The model under review builds one solid part; all positions refer to its coordinate system, in mm. A direction names the side the tool comes from. Round coordinates to 2 decimals unless told otherwise and drop trailing zeros. Order: outer loops, then holes, each group sorted by start corner. A loop starts at its lowest first (then second) coordinate and runs counter-clockwise, first axis right, second up.
1) Consider section A-A (z = -3.2). Give the boundary of the cut face in (x, y).
2) Mouldability with a two-part tool opening along X and no side actions: class faces 1 (the face through (6.506, 0.072, -0.986)), 2 (the face through (-17.922, -9.404, -2.416)), 3 (the face through (-14, -9, -4)) as pulls with the +X half, pulls with the -X half, needs draft (parallel to the pull), parting line crosses it, or undercut.
3) Clearance check with flat-ended pins moving along their axes: P1, Ø1.5, axis at x = 4.5, z = -3, coming from the +Y side; P2, Ø12, axis at x = -6.5, y = 8, coming from the -Z side; P3, Ø1.5, axis at y = 0.5, z = -1, coming from the -X side. State where each tip first meets the part, or that it passes through.
4) Consider section D-D (x = -2). Give the boundary of the cut face in (y, z).
5) Consider section B-B (y = 7.7). Give the boundary of the cut face in (x, z).
6) Machinability: for faces 4 (the face through (6, -4.9, -1)), 5 (the face through (18.286, 6.628, -2.416)), 6 (the face through (0, -10.5, -1)), 7 (the face through (-6, 4.9, -1)), which of the approach directions +Z, -Z, +X, -X, +Y, -Y give a long, thin tool a straight path to every point of the face, cutting with its end or side? Answer none if there is none.
7) To check wall thickness, follow L1, parallel to Y at x = 15.7, z = -2.7; L2, parallel to Y at x = -15.7, z = -2.5; L3, parallel to Z at x = -2, y = 0.5. State the ranges of each line that lie inside material, in increasing order.
8) Consider section C-C (x = 11). Give the boundary of the cut face in (y, z).
from build123d import *

# Parameters (mm, degrees)
EXTRUDE_1007_DEPTH = 2
SKETCH_1_5_R       = 2.8
SKETCH_1_5_R_2     = 1.7
EXTRUDE_1109_DEPTH = 4


with BuildPart() as part:
    # Эскиз1 → Extrude 1007 (new body)
    with BuildSketch(Plane.XY):
        with BuildLine():
            Line((15.7, 10.5), (-15.7, 10.5))
            ThreePointArc((-15.7, 10.5), (-13.720101013, 9.679898987), (-12.9, 7.7))
            ThreePointArc((-12.9, 7.7), (-13.720101013, 5.720101013), (-15.7, 4.9))
            Line((-15.7, 4.9), (3.632157719, 4.9))
            Line((3.632157719, 4.9), (-16.932946461, -5.186070203))
            ThreePointArc((-16.932946461, -5.186070203), (-14.218826494, -5.323842378), (-12.9, -7.7))
            ThreePointArc((-12.9, -7.7), (-13.720101013, -9.679898987), (-15.7, -10.5))
            Line((-15.7, -10.5), (15.7, -10.5))
            ThreePointArc((15.7, -10.5), (12.9, -7.7), (15.7, -4.9))
            Line((15.7, -4.9), (-3.632157719, -4.9))
            Line((-3.632157719, -4.9), (16.932946461, 5.186070203))
            ThreePointArc((16.932946461, 5.186070203), (12.972455002, 7.067150662), (15.7, 10.5))
        make_face()
    extrude(amount=-EXTRUDE_1007_DEPTH)

    # Эскиз1<5> → Extrude 1109 (add)
    # profile 1 of 4: a face of its own
    with BuildSketch(Plane.XY):
        with Locations((15.7, 7.7)):
            Circle(SKETCH_1_5_R)
        with Locations((15.7, 7.7)):
            Circle(SKETCH_1_5_R_2, mode=Mode.SUBTRACT)
    # profile 2 of 4: a face of its own
    with BuildSketch(Plane.XY):
        with Locations((15.7, -7.7)):
            Circle(SKETCH_1_5_R)
    # profile 3 of 4: a face of its own
    with BuildSketch(Plane.XY):
        with Locations((-15.7, -7.7)):
            Circle(SKETCH_1_5_R)
        with Locations((-15.7, -7.7)):
            Circle(SKETCH_1_5_R_2, mode=Mode.SUBTRACT)
    # profile 4 of 4: a face of its own
    with BuildSketch(Plane.XY):
        with Locations((-15.7, 7.7)):
            Circle(SKETCH_1_5_R)
    extrude(amount=-EXTRUDE_1109_DEPTH)


solid = part.part
Answer below:
1. outline: circle Ø5.6 at (-15.7, -7.7); circle Ø5.6 at (-15.7, 7.7); circle Ø5.6 at (15.7, -7.7); circle Ø5.6 at (15.7, 7.7); hole circle Ø3.4 at (-15.7, -7.7); hole circle Ø3.4 at (15.7, 7.7)
2. face 1: pulls with the +X half
2. face 2: undercut
2. face 3: needs draft
3. P1: passes through
3. P2: stops at z = -2
3. P3: stops at x = -6.87
4. outline: (-10.5, -2) - (-4.9, -2) - (-4.9, 0) - (-10.5, 0) - close; (-4.1, -2) - (2.14, -2) - (2.14, 0) - (-4.1, 0) - close; (4.9, -2) - (10.5, -2) - (10.5, 0) - (4.9, 0) - close
5. outline: (-18.5, -4) - (-12.9, -4) - (-12.9, -2) - (12.9, -2) - (12.9, -4) - (14, -4) - (14, 0) - (-18.5, 0) - close; (17.4, -4) - (18.5, -4) - (18.5, 0) - (17.4, 0) - close
6. face 4: +Z, -Z, +X
6. face 5: -Z
6. face 6: +Z, -Z, +X, -X, -Y
6. face 7: +Z, -Z, -X
7. L1: y = -10.5 to -4.9, 4.9 to 6, 9.4 to 10.5
7. L2: y = -10.5 to -9.4, -6 to -4.9, 4.9 to 10.5
7. L3: z = -2 to 0
8. outline: (-10.5, -2) - (-4.9, -2) - (-4.9, 0) - (-10.5, 0) - close; (2.28, -2) - (10.5, -2) - (10.5, 0) - (2.28, 0) - close
